For this review, take the finished solid that the model builds, in its own axes (mm). A direction names the side the tool comes from. Give positions to 0.01 mm unless a question says otherwise; leave off trailing zeros. Loops run counter-clockwise (first coordinate to the right, second up) from the corner with the lowest first, then second, coordinate; pieces in that order, holes last. Notation, with made-up numbers: (-27.5, 65) - (4.5, 65) arc R9 ccw to (4.5, 76) - close; hole circle Ø10 at (-7, 61). An arc over 180 degrees is marked (long way). Use CSV: the item, a comma, the result in double quotes. Start each with the question number.
1. For faces 1 (the flat face through (0, -25.4, 0)), 2 (the flat face through (0, -76.2, -8)), list the 3-axis set-ups (+Z, -Z, +X, -X, +Y, -Y) from which the entire face can be reached by the end or side of a thin tool; tool diameter is ignored.
2. Take a section at B-B on x = 0. Give the boundary of the cut face in (y, z).
3. Take a section at A-A on z = 0. Give the boundary of the cut face in (x, y), plus the area to 3 significant figures.
4. For pin 1 (2 mm diameter, centred on x = 11.5, y = -17, fed in from -Z); pin 2 (10 mm diameter, centred on x = -13, y = -58, fed in from +Z); pin 3 (6 mm diameter, centred on y = -47, z = 16.5, fed in from +X), all flat-tipped, find the tip position at first contact; note any pin that passes through.
5. Take a section at C-C on y = -47.5. Give the boundary of the cut face in (x, z).
6. Wall thickness on line 1 (Z direction, x = 0, y = -46); line 2 (Y direction, x = 7, z = -0.5); line 3 (Z direction, x = 3.5, y = -48): over which ranges is each line inside the solid? List them lowest first.
7. Mouldability with a two-part tool opening along X and no side actions: class faces 3 (the cylindrical face through (-5.77, -51.16, -4.42)), 4 (the flat face through (0, 0, 0)), 5 (the cylindrical face through (23.24, -32.49, 7.32)) as pulls with the +X half, pulls with the -X half, needs draft (parallel to the pull), parting line crosses it, or undercut.
```python
from build123d import *

# Parameters (mm, degrees)
F0_R     = 24.3653753529
F1_DEPTH = 76.2
F2_R     = 7.62
F3_R     = 7.2684002017
F4_DEPTH = 50.8
F5_SIZE2 = 18.1374796856
F5_SIZE  = 12.7


with BuildPart() as f1:
    # F0 (on Front) → F1 (new body)
    with BuildSketch(Plane.XZ):
        Circle(F0_R)
    extrude(amount=F1_DEPTH)

    # F2
    f2_edges = [f1.edges().sort_by_distance(p)[0] for p in [
        (-24.365375, 0, 0),
    ]]
    fillet(f2_edges, radius=F2_R)

    # F3 (on face) → F4 (cut)
    with BuildSketch(Plane.XZ.offset(76.2)):
        Circle(F3_R)
    extrude(amount=-F4_DEPTH, mode=Mode.SUBTRACT)

    # F5
    f5_edges = [f1.edges().sort_by_distance(p)[0] for p in [
        (-24.365375, -76.2, 0),
    ]]
    f5_side = f1.faces().sort_by_distance((-23.676218, -76.2, 0))[0]
    chamfer(f5_edges, length=F5_SIZE, length2=F5_SIZE2, reference=f5_side)


solid = f1.part
```
Check result:
1,face 1,"-Y"
1,face 2,"+Z, -Z, +X, -X, -Y"
2,outline,"(-76.2, -11.67) - (-58.06, -24.37) - (-7.62, -24.37) arc R7.62 ccw to (0, -16.75) - (0, 16.75) arc R7.62 ccw to (-7.62, 24.37) - (-58.06, 24.37) - (-76.2, 11.67) - (-76.2, 7.27) - (-25.4, 7.27) - (-25.4, -7.27) - (-76.2, -7.27) - close"
3,outline,"(-24.37, -58.06) - (-11.67, -76.2) - (-7.27, -76.2) - (-7.27, -25.4) - (7.27, -25.4) - (7.27, -76.2) - (11.67, -76.2) - (24.37, -58.06) - (24.37, -7.62) arc R7.62 ccw to (16.75, 0) - (-16.75, 0) arc R7.62 ccw to (-24.37, -7.62) - close"
3,area,"2,720 mm²"
4,pin 1,"stops at z = -21.99"
4,pin 2,"stops at z = 23.01"
4,pin 3,"stops at x = 20.28"
5,outline,"circle Ø48.73 at (0, 0); hole circle Ø14.54 at (0, 0)"
6,line 1,"z = -24.37 to -7.27, 7.27 to 24.37"
6,line 2,"y = -25.4 to 0"
6,line 3,"z = -24.11 to -6.37, 6.37 to 24.11"
7,face 3,"undercut"
7,face 4,"needs draft"
7,face 5,"parting line crosses it"
